```python
from build123d import *

# Parameters (mm, degrees)
BOSS_EXTRUDE1_DEPTH = 75.819


with BuildPart() as part:
    # Sketch1 → Boss-Extrude1 (new, symmetric)
    with BuildSketch(Plane.XY):
        with BuildLine():
            Line((-19.05, -41.467593741), (-8.981837469, -34.152645484))
            ThreePointArc((-8.981837469, -34.152645484), (9.380639725, -37.883478952), (19.812, -22.317926926))
            Line((19.812, -22.317926926), (19.812, -19.777926926))
            ThreePointArc((19.812, -19.777926926), (11.176, -23.166133114), (2.54, -19.777926926))
            Line((2.54, -19.777926926), (0, -19.777926926))
            Line((0, -19.777926926), (-25.4, -38.232107137))
            Line((-25.4, -38.232107137), (-25.4, -79.567593741))
            Line((-25.4, -79.567593741), (-19.05, -79.567593741))
            Line((-19.05, -79.567593741), (-19.05, -41.467593741))
        make_face()
    extrude(amount=BOSS_EXTRUDE1_DEPTH, both=True)

    # Sketch2 → Revolve1 (revolve)
    with BuildSketch(Plane.XY.offset(75.819)):
        with BuildLine():
            Line((1.27, -20.412926926), (1.27, -24.222926926))
            ThreePointArc((1.27, -24.222926926), (3.175, -22.317926926), (1.27, -20.412926926))
        make_face()
    revolve(axis=Axis((1.27, -20.412926926, 75.819), (0, -1, 0)))

    # Sketch3 → Revolve2 (revolve)
    with BuildSketch(Plane(origin=(0, 0, -75.819), x_dir=(-1, 0, 0), z_dir=(0, 0, -1))):
        with BuildLine():
            Line((-1.27, -20.412926926), (-1.27, -24.222926926))
            ThreePointArc((-1.27, -24.222926926), (0.635, -22.317926926), (-1.27, -20.412926926))
        make_face()
    revolve(axis=Axis((1.27, -20.412926926, -75.819), (0, -1, 0)))


solid = part.part
```
Verification items for the finished model (mm, model axes). A direction names the side the tool comes from. Round coordinates to 2 decimals unless told otherwise and drop trailing zeros. Write each loop counter-clockwise with the first axis right and the second up, starting at its lowest first coordinate (ties: lowest second). Pieces come first, ordered by that corner, then holes. Notation, with made-up numbers: (33.25, 67) - (90.25, 67) arc R14 cw to (90.25, 88) - close; hole circle Ø10 at (64, 49.25). An arc over 180 degrees is marked (long way). Answer as a JSON object with one key per item and string values. Group by question number.
Q1. Section check A-A, the plane z = 22. Enter the section's corners in (x, y).
Q2. Section check B-B, the plane y = -61. Enter the section's corners in (x, z), plus the area to 3 significant figures.
Q3. Go/stop test with flat-tipped pins: pin 1 Ø19 at (y, z) = (-57.5, -28) entering from +X; pin 2 Ø13.5 at (x, y) = (-14, -50) entering from -Z; pin 3 Ø8 at (x, z) = (-16, 19) entering from +Y. Record where each tip stops, or that it passes through.
Q4. Mould release check, pull along X, two halves, no side actions. Record for faces 1 (the flat face through (-25.4, -59, 1)), 2 (the cylindrical face through (11.309, -23.165, 1.061)), 3 (the flat face through (-19.05, -61, 1)), 4 (the cylindrical face through (9.12, -37.99, 1.06)): released by +X, released by -X, zero draft, split by the parting line, or undercut.
Q5. Thickness scan on line 1 (Z direction, x = -22, y = -55.5); line 2 (X direction, y = -59, z = 30); line 3 (X direction, y = -35.5, z = -67). Record the ranges inside material, lowest first.
Q6. Tool access check on faces 5 (the flat face through (-14.086, -37.861, 1.061)), 6 (the flat face through (-12.522, -28.876, 1.061)). Record the directions out of +Z, -Z, +X, -X, +Y, -Y that give a thin tool (end or side, any length) a straight path to the whole face; none if there is none.
Q7. Section check C-C, the plane x = 17.5. Enter the section's corners in (y, z), plus the area to 3 significant figures.
Found:
{
 "1": {"outline": "(-25.4, -79.57) - (-19.05, -79.57) - (-19.05, -41.47) - (-8.98, -34.15) arc R16.83 ccw to (19.81, -22.32) - (19.81, -19.78) arc R12.7 cw to (2.54, -19.78) - (0, -19.78) - (-25.4, -38.23) - close"},
 "2": {"outline": "(-25.4, -75.82) - (-19.05, -75.82) - (-19.05, 75.82) - (-25.4, 75.82) - close", "area": "963 mm^2"},
 "3": {"pin 1": "stops at x = -19.05", "pin 2": "stops at z = -75.82", "pin 3": "stops at y = -28.5"},
 "4": {"face 1": "released by -X", "face 2": "undercut", "face 3": "released by +X", "face 4": "undercut"},
 "5": {"line 1": "z = -75.82 to 75.82", "line 2": "x = -25.4 to -19.05", "line 3": "x = -21.64 to -10.84, -7.48 to 13.44"},
 "6": {"face 5": "+Z, -Z, -Y", "face 6": "+Z, -Z, -X, +Y"},
 "7": {"outline": "(-30.83, -75.82) - (-21.48, -75.82) - (-21.48, 75.82) - (-30.83, 75.82) - close", "area": "1,420 mm^2"}
}
